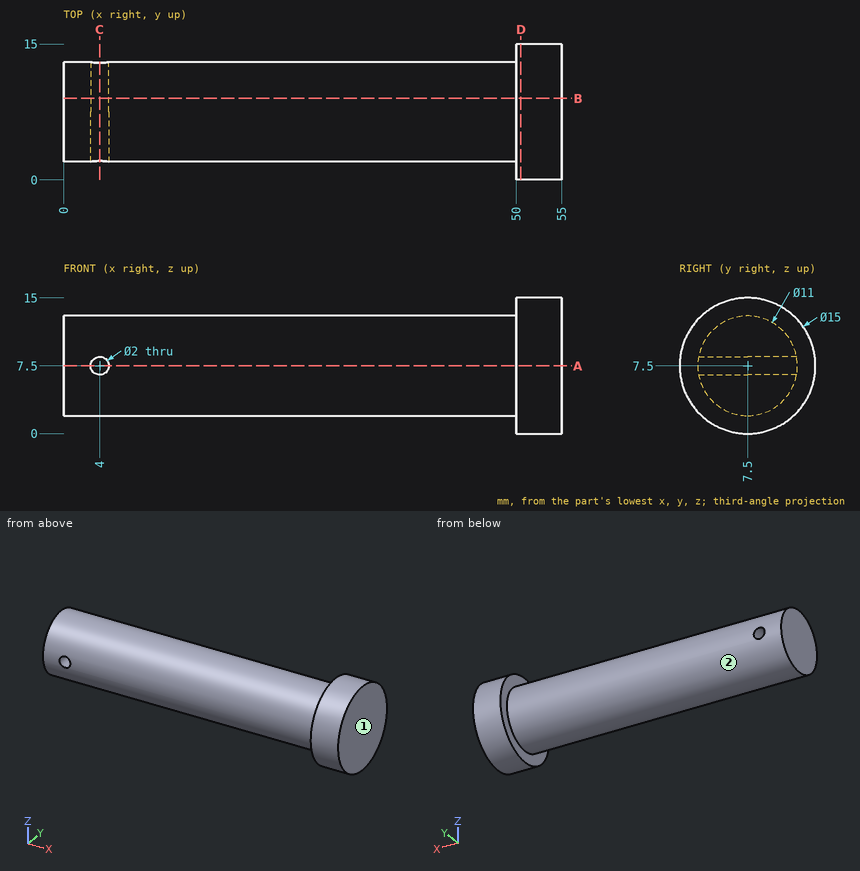
Part print with two shaded views. Sizes in mm from the minimum x, y, z corner. A direction names the side the tool comes from. Round coordinates to 2 decimals unless told otherwise and drop trailing zeros. Write each loop counter-clockwise with the first axis right and the second up, starting at its lowest first coordinate (ties: lowest second). Pieces come first, ordered by that corner, then holes. Notation, with made-up numbers: M 68.25,61 L 124.25,61 A8 cw 124.25,73 Z; hole C 34.25,74.25 d4. An arc over 180 degrees is marked long. Put each result on its own line as item: value. Start each with the question number.
1) 3-axis set-ups, long thin cutter, end or side, ignore diameter. For the marked faces 1 and 2: which of +Z, -Z, +X, -X, +Y, -Y reach the whole face in a straight line?
2) Saw through at A-A, the plane z = 7.5. Write the cut outline in (x, y).
3) Saw through at B-B, the plane y = 9. Write the cut outline in (x, z).
4) Saw through at C-C, the plane x = 4. Write the cut outline in (y, z), and give its area (3 significant figures).
5) Drill centre lines: probe 1 along X at (y, z) = (4.9, 7.5); probe 2 along X at (y, z) = (8.25, 1); probe 3 along Z at (x, y) = (51, 7.25). Where is each one in solid material? Low to high. Write a range as [from, to].
6) Pin check, flat tips, straight feed: pin 1 Ø4 at (x, z) = (24.5, 3) entering from +Y; pin 2 Ø5 at (x, z) = (11, 6) entering from -Y; pin 3 Ø3 at (x, y) = (19.5, 6.5) entering from -Z. Stop position of each tip, or through.
7) Saw through at D-D, the plane x = 50.5. Write the cut outline in (y, z), and give its area (3 significant figures).
Resolved:
1. face 1: +Z, -Z, +X, +Y, -Y
1. face 2: -X
2. outline: M 0,2 L 3,2 L 3,13 L 0,13 Z; M 5,2 L 50,2 L 50,0 L 55,0 L 55,15 L 50,15 L 50,13 L 5,13 Z
3. outline: M 0,2.21 L 50,2.21 L 50,0.15 L 55,0.15 L 55,14.85 L 50,14.85 L 50,12.79 L 0,12.79 Z; hole C 4,7.5 d2
4. outline: M 2.09,6.5 A5.5 ccw 12.91,6.5 Z; M 2.09,8.5 L 12.91,8.5 A5.5 ccw Z
4. area: 73.2 mm²
5. probe 1: [0, 3], [5, 55]
5. probe 2: [50, 55]
5. probe 3: [0, 15]
6. pin 1: y = 12.4
6. pin 2: y = 2
6. pin 3: z = 2
7. outline: C 7.5,7.5 d15
7. area: 177 mm²
